Source: CAD feature listing. Evaluate the final solid. Frame: model axes, mm. Face numbers are marked on the shaded views. Round coordinates to 2 decimals unless told otherwise and drop trailing zeros. Write each loop counter-clockwise with the first axis right and the second up, starting at its lowest first coordinate (ties: lowest second). Pieces come first, ordered by that corner, then holes. Notation, with made-up numbers: M 11.25,82 L 42.25,82 A19 cw 42.25,88 Z; hole C 84.25,14 d5. An arc over 180 degrees is marked long. Put each result on its own line as item: value. Start each with the question number.
```python
from build123d import *

# Parameters (mm, degrees)
SKETCH1_W            = 145.7
SKETCH1_H            = 45
BOSS_EXTRUDE1_DEPTH  = 2
SKETCH17_W           = 145.7
SKETCH17_H           = 45
SKETCH17_W_2         = 140.7
SKETCH17_H_2         = 40
SKETCH17_W_3         = 139.5
SKETCH17_H_3         = 38.8
SKETCH17_W_4         = 137.1
SKETCH17_H_4         = 36.4
BOSS_EXTRUDE10_DEPTH = 5
FILLET2_R            = 2


with BuildPart() as part:
    # Sketch1 → Boss-Extrude1 (new body)
    with BuildSketch(Plane.XY):
        with Locations((72.85, 22.5)):
            Rectangle(SKETCH1_W, SKETCH1_H)
    extrude(amount=BOSS_EXTRUDE1_DEPTH)

    # Sketch17 → Boss-Extrude10 (add)
    # profile 1 of 2: a face of its own
    with BuildSketch(Plane.XY.offset(2)):
        with Locations((72.85, 22.5)):
            Rectangle(SKETCH17_W, SKETCH17_H)
        with Locations((72.85, 22.5)):
            Rectangle(SKETCH17_W_2, SKETCH17_H_2, mode=Mode.SUBTRACT)
    # profile 2 of 2: a face of its own
    with BuildSketch(Plane.XY.offset(2)):
        with Locations((72.85, 22.5)):
            Rectangle(SKETCH17_W_3, SKETCH17_H_3)
        with Locations((72.85, 22.5)):
            Rectangle(SKETCH17_W_4, SKETCH17_H_4, mode=Mode.SUBTRACT)
    extrude(amount=BOSS_EXTRUDE10_DEPTH)

    # Fillet2
    fillet2_edges = [part.edges().sort_by_distance(p)[0] for p in [
        (0, 45, 3.5),
        (145.7, 45, 3.5),
        (145.7, 0, 3.5),
        (0, 0, 3.5),
    ]]
    fillet(fillet2_edges, radius=FILLET2_R)


solid = part.part
```
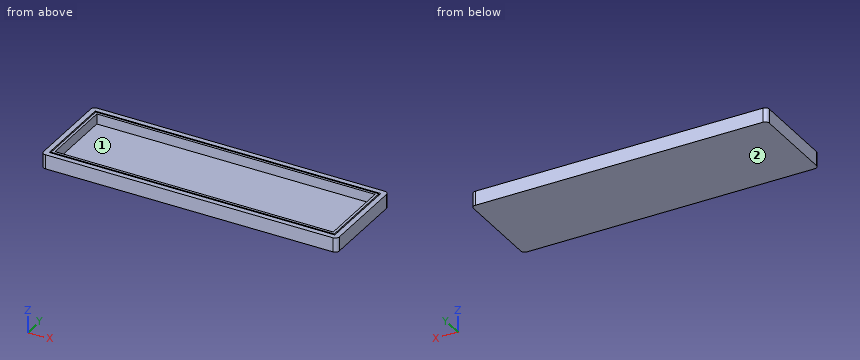
(1) Ray query, line 1 along Y through (x, z) = (16.5, 2.25); line 2 along X through (y, z) = (41.5, 3.75); line 3 along X through (y, z) = (40, 5.5). Return the intervals inside material, ascending.
(2) Pull-direction query (X, two-part tool) for the marked faces 1 and 2; classes: +X half, -X half, draft (parallel to the pull), parting line (faces both ways), or undercut.
(3) Section query A-A (z = 3.25). Return loops of the section in (x, y).
(4) Contact query for flat-ended pins moving along their axis: P1, Ø10, axis at x = 86.5, y = 30.5, coming from the -Z side; P2, Ø8, axis at x = 17.5, y = 17.5, coming from the +Z side. Output: stop coordinate, or through.
(5) Section query C-C (y = 12.5). Return loops of the section in (x, z), and give its area (3 significant figures).
(6) Section query B-B (x = 101.5). Return loops of the section in (y, z).
Entries:
1. line 1: 0 to 2.5, 3.1 to 4.3, 40.7 to 41.9, 42.5 to 45
1. line 2: 0 to 2.5, 3.1 to 142.6, 143.2 to 145.7
1. line 3: 0 to 2.5, 3.1 to 4.3, 141.4 to 142.6, 143.2 to 145.7
2. face 1: undercut
2. face 2: draft
3. outline: M 0,2 A2 ccw 2,0 L 143.7,0 A2 ccw 145.7,2 L 145.7,43 A2 ccw 143.7,45 L 2,45 A2 ccw 0,43 Z; M 3.1,3.1 L 142.6,3.1 L 142.6,41.9 L 3.1,41.9 Z; hole M 2.5,2.5 L 143.2,2.5 L 143.2,42.5 L 2.5,42.5 Z; hole M 4.3,4.3 L 141.4,4.3 L 141.4,40.7 L 4.3,40.7 Z
4. P1: z = 0
4. P2: z = 2
5. outline: M 0,0 L 145.7,0 L 145.7,7 L 143.2,7 L 143.2,2 L 142.6,2 L 142.6,7 L 141.4,7 L 141.4,2 L 4.3,2 L 4.3,7 L 3.1,7 L 3.1,2 L 2.5,2 L 2.5,7 L 0,7 Z
5. area: 328 mm2
6. outline: M 0,0 L 45,0 L 45,7 L 42.5,7 L 42.5,2 L 41.9,2 L 41.9,7 L 40.7,7 L 40.7,2 L 4.3,2 L 4.3,7 L 3.1,7 L 3.1,2 L 2.5,2 L 2.5,7 L 0,7 Z
